Geometry check sheet. Reference: the model listing, model coordinates, mm. A direction names the side the tool comes from. Give positions to 0.01 mm unless a question says otherwise; leave off trailing zeros. Write each loop counter-clockwise with the first axis right and the second up, starting at its lowest first coordinate (ties: lowest second). Pieces come first, ordered by that corner, then holes. Notation, with made-up numbers: M 57.25,-15.75 L 105.25,-15.75 A9 cw 105.25,0.25 Z; hole C 47,34.25 d5. An arc over 180 degrees is marked long. Use one line per item in the form item = value. Start each with the question number.
```python
from build123d import *

# Parameters (mm, degrees)
SKETCH_1_W          = 8
SKETCH_1_H          = 8
EXTRUDE_1_DEPTH     = 20
SKETCH_2_R          = 1.8
CUT_EXTRUDE_1_DEPTH = 23.978250586
SKETCH_4_W          = 2
SKETCH_4_H          = 8
EXTRUDE_3_DEPTH     = 10
SKETCH_5_W          = 5.2
SKETCH_5_H          = 8.5
CUT_EXTRUDE_2_DEPTH = 24.748684174
FILLET_1_R          = 3
SKETCH_6_R          = 1.45
CUT_EXTRUDE_3_DEPTH = 25.657656012
FILLET_2_R          = 3


with BuildPart() as part:
    # 草图1 → 凸台-拉伸1 (new body)
    with BuildSketch(Plane(origin=(0, 0, 0), x_dir=(1, 0, 0), z_dir=(0, 1, 0))):
        with Locations((4, -4)):
            Rectangle(SKETCH_1_W, SKETCH_1_H)
    extrude(amount=EXTRUDE_1_DEPTH)

    # 草图2 → 切除-拉伸1 (cut, through all)
    with BuildSketch(Plane.XY.offset(8)):
        with Locations((4, 4)):
            Circle(SKETCH_2_R)
    extrude(amount=-CUT_EXTRUDE_1_DEPTH, mode=Mode.SUBTRACT)

    # 草图4 → 凸台-拉伸3 (add)
    with BuildSketch(Plane(origin=(0, 20, 0), x_dir=(1, 0, 0), z_dir=(0, 1, 0))):
        with Locations((-1, -4)):
            Rectangle(SKETCH_4_W, SKETCH_4_H)
        with Locations((9, -4)):
            Rectangle(SKETCH_4_W, SKETCH_4_H)
    extrude(amount=-EXTRUDE_3_DEPTH)

    # 草图5 → 切除-拉伸2 (cut, through all)
    with BuildSketch(Plane.XY.offset(8)):
        with Locations((4, 15.75)):
            Rectangle(SKETCH_5_W, SKETCH_5_H)
    extrude(amount=-CUT_EXTRUDE_2_DEPTH, mode=Mode.SUBTRACT)

    # 圆角1
    # the kernel refuses this fillet: 3 mm, written as the material it adds along each edge
    with BuildSketch(Plane(origin=(8, 10, 8), x_dir=(0, -1, 0), z_dir=(0, 0, -1))) as fillet_1_piece_1:
        with BuildLine():
            CenterArc((2.828427125, -3), FILLET_1_R, 90, 70.528779366)
            Line((0, -2), (-0.056568542, -1.98))
            ThreePointArc((-0.056568542, -1.98), (-0.06, -1), (-0.06, 0))
            Line((-0.06, 0), (0, 0.06))
            Line((0, 0.06), (2.828427125, 0.06))
            Line((2.828427125, 0.06), (2.828427125, 0))
        make_face()
    extrude(amount=8)
    with BuildSketch(Plane(origin=(0, 10, 8), x_dir=(-1, 0, 0), z_dir=(0, 0, -1))) as fillet_1_piece_2:
        with BuildLine():
            CenterArc((3, -2.828427125), FILLET_1_R, 109.471220634, 70.528779366)
            Line((0, -2.828427125), (-0.06, -2.828427125))
            Line((-0.06, -2.828427125), (-0.06, 0))
            Line((-0.06, 0), (0, 0.06))
            ThreePointArc((0, 0.06), (1, 0.06), (1.98, 0.056568542))
            Line((1.98, 0.056568542), (2, 0))
        make_face()
    extrude(amount=8)

    # 草图6 → 切除-拉伸3 (cut, through all)
    with BuildSketch(Plane(origin=(10, 0, 0), x_dir=(0, 0, -1), z_dir=(1, 0, 0))):
        with Locations((-4, 16)):
            Circle(SKETCH_6_R)
    extrude(amount=-CUT_EXTRUDE_3_DEPTH, mode=Mode.SUBTRACT)

    # 圆角2
    fillet_2_edges = [part.edges().sort_by_distance(p)[0] for p in [
        (8.3, 20, 0),
        (-2, 10, 4),
        (10, 10, 4),
        (-0.3, 20, 0),
        (8.3, 20, 8),
        (8, 0, 4),
        (0, 0, 4),
        (-0.3, 20, 8),
    ]]
    fillet(fillet_2_edges, radius=FILLET_2_R)


solid = part.part
```
(1) Sectioned sample at B-B, the plane y = 4. Record the boundary of the cut face in (x, z), plus the area to 3 significant figures.
(2) Sectioned sample at D-D, the plane y = 16. Record the boundary of the cut face in (x, z), plus the area to 3 significant figures.
(3) Thickness scan on probe 1 along Y at (x, z) = (4, 4.5); probe 2 along X at (y, z) = (11.75, 2); probe 3 along X at (y, z) = (6, 3.5). Record the ranges inside material, lowest first. Write a range as [from, to].
(4) Draft check along X on faces 1 (the cylindrical face through (8.32, 19.1, 0.86)), 2 (the flat face through (10, 14, 4)), 3 (the cylindrical face through (5.717, 4.541, 4.056)), 4 (the flat face through (4, 11.5, 4)). Enter one of: released by +X, released by -X, zero draft, split by the parting line, or undercut.
(5) Sectioned sample at A-A, the plane z = 4. Record the boundary of the cut face in (x, y), plus the area to 3 significant figures.
(6) Depth check by flat-ended pin: pin 1 (2.5 mm diameter, centred on x = 4, z = 3.5, fed in from +Y); pin 2 (4.5 mm diameter, centred on y = 4, z = 3.5, fed in from +X); pin 3 (2 mm diameter, centred on y = 5, z = 2, fed in from -X). Enter the tip coordinate at first touch or a pass-through.
(7) Tool access check on faces 5 (the flat face through (0, 5, 4)), 6 (the flat face through (1.4, 14, 4)), 7 (the flat face through (-2, 14, 4)). Record the directions out of +Z, -Z, +X, -X, +Y, -Y that give a thin tool (end or side, any length) a straight path to the whole face; none if there is none.
(8) Sectioned sample at C-C, the plane x = 4. Record the boundary of the cut face in (y, z), plus the area to 3 significant figures.
Numbers:
q1.outline = M 0,0 L 2.2,0 L 2.2,8 L 0,8 Z; M 5.8,0 L 8,0 L 8,8 L 5.8,8 Z
q1.area = 35.2 mm2
q2.outline = M -2,0 L 1.4,0 L 1.4,2.55 L -2,2.55 Z; M -2,5.45 L 1.4,5.45 L 1.4,8 L -2,8 Z; M 6.6,0 L 10,0 L 10,2.55 L 6.6,2.55 Z; M 6.6,5.45 L 10,5.45 L 10,8 L 6.6,8 Z
q2.area = 34.7 mm2
q3.probe_1 = [0, 2.2], [5.8, 11.5]
q3.probe_2 = [-2, 1.4], [6.6, 10]
q3.probe_3 = [0, 8]
q4.face_1 = zero draft
q4.face_2 = released by +X
q4.face_3 = undercut
q4.face_4 = undercut
q5.outline = M -2,11.64 A3 ccw -1,9.41 A3 cw 0,7.17 L 0,3 A3 ccw 3,0 L 5,0 A3 ccw 8,3 L 8,7.17 A3 cw 9,9.41 A3 ccw 10,11.64 L 10,14.55 L 6.6,14.55 L 6.6,11.5 L 1.4,11.5 L 1.4,14.55 L -2,14.55 Z; M -2,17.45 L 1.4,17.45 L 1.4,20 L -2,20 Z; M 6.6,17.45 L 10,17.45 L 10,20 L 6.6,20 Z; hole C 4,4 d3.6
q5.area = 124 mm2
q6.pin_1 = 11.5
q6.pin_2 = 8
q6.pin_3 = 0
q7.face_5 = +Z, -Z, -X, -Y
q7.face_6 = +Z, -Z, +Y
q7.face_7 = +Z, -Z, -X, +Y, -Y
q8.outline = M 0,0 L 2.2,0 L 2.2,8 L 0,8 Z; M 5.8,0 L 11.5,0 L 11.5,8 L 5.8,8 Z
q8.area = 63.2 mm2
